```python
from build123d import *

# Parameters (mm, degrees)
SKETCH1_R           = 3.429
BOSS_EXTRUDE1_DEPTH = 6.35


with BuildPart() as part:
    # Sketch1 → Boss-Extrude1 (new body)
    with BuildSketch(Plane(origin=(0, 0, 0), x_dir=(1, 0, 0), z_dir=(0, 1, 0))):
        Polygon((-189.09320701, -158.66804026), (-280.551178696, -202.917327431), (-457.2, -58.822791946), (-457.2, 0), (0, 0), align=None)
        with Locations((-207.494657953, -160.516879503)):
            Circle(SKETCH1_R, mode=Mode.SUBTRACT)
        with Locations((-276.088136717, -193.703844882)):
            Circle(SKETCH1_R, mode=Mode.SUBTRACT)
        with Locations((-57.15, -7.62)):
            Circle(SKETCH1_R, mode=Mode.SUBTRACT)
        with Locations((-379.73, -7.62)):
            Circle(SKETCH1_R, mode=Mode.SUBTRACT)
    extrude(amount=BOSS_EXTRUDE1_DEPTH)


solid = part.part
```
Work out the finished part from the listing and answer in its coordinate system (mm). Give positions to 0.01 mm unless a question says otherwise; leave off trailing zeros. Write each loop counter-clockwise with the first axis right and the second up, starting at its lowest first coordinate (ties: lowest second). Pieces come first, ordered by that corner, then holes. Notation, with made-up numbers: (85, -28) - (118, -28) arc R34 cw to (118, 6) - close; hole circle Ø8 at (11, -32). An arc over 180 degrees is marked (long way). Use one line per item in the form item = value.
1. Consider L1, parallel to X at y = 2.25, z = 7.62; L2, parallel to Z at x = -368, y = 3.25; L3, parallel to X at y = 5.25, z = 119. Determine where each line is inside the solid, lowest interval first.
Filled in:
L1 = -457.2 to -383.16, -376.3 to -60.58, -53.72 to -9.08
L2 = 0 to 131.58
L3 = -383.43 to -141.82
2. A cutting plane is placed at A-A (y = 3). Write down the section's boundary in (x, z), and give its area (3 significant figures).
Filled in:
outline = (-457.2, 0) - (0, 0) - (-189.09, 158.67) - (-280.55, 202.92) - (-457.2, 58.82) - close; hole circle Ø6.86 at (-379.73, 7.62); hole circle Ø6.86 at (-276.09, 193.7); hole circle Ø6.86 at (-207.49, 160.52); hole circle Ø6.86 at (-57.15, 7.62)
area = 54,500 mm^2
3. Determine the mould class of faces 1 (the face through (-93.22, 3.13, 78.22)), 2 (the face through (-225, 6.35, 77)), 3 (the face through (-225, 0, 77)) for opening direction Y: released by +Y, released by -Y, zero draft, split by the parting line, or undercut.
Filled in:
face_1 = zero draft
face_2 = released by +Y
face_3 = released by -Y
4. A cutting plane is placed at C-C (x = -178). Write down the section's boundary in (y, z), and give its area (3 significant figures).
Filled in:
outline = (0, 0) - (6.35, 0) - (6.35, 149.36) - (0, 149.36) - close
area = 948 mm^2
5. A cutting plane is placed at B-B (z = 143). Write down the section's boundary in (x, y), and give its area (3 significant figures).
Filled in:
outline = (-354.01, 0) - (-170.42, 0) - (-170.42, 6.35) - (-354.01, 6.35) - close
area = 1,170 mm^2
6. Each of these flat-tipped pins is pushed along its axis until it touches: pin 1 Ø3 at (x, y) = (-69, 3.5) entering from -Z; pin 2 Ø1.5 at (x, y) = (-97, 5) entering from +Z. Where does it stop, or does it pass through?
Filled in:
pin_1 = 0
pin_2 = 82.02
